Input: part model. Units: mm. Frame: model coordinates. Coordinates: 2 decimals unless noted, no trailing zeros. Write each loop counter-clockwise with the first axis right and the second up, starting at its lowest first coordinate (ties: lowest second). Pieces come first, ordered by that corner, then holes. Notation, with made-up numbers: (-22, -27) -> (35, -27) arc R16 ccw to (35, -22) -> close; hole circle Ø11 at (75.5, -38). An arc over 180 degrees is marked (long way). Use one line per item in the form item = value. Start each with the question number.
(1) Cut plane C-C on y = 0.8. State how many separate pieces and enclosed holes the cut face has, plus the area to 4 significant figures.
(2) Cut plane B-B on z = 8. Return the cut outline in (x, y) (3 decimals).
(3) Ray query, line 1 along X through (y, z) = (0.85, 160); line 2 along Z through (x, y) = (2.5, 0.6); line 3 along X through (y, z) = (1.55, 100). Return the intervals inside material, ascending.
(4) Cut plane A-A on x = 48. Return the cut outline in (y, z) (3 decimals), plus the area to 3 significant figures.
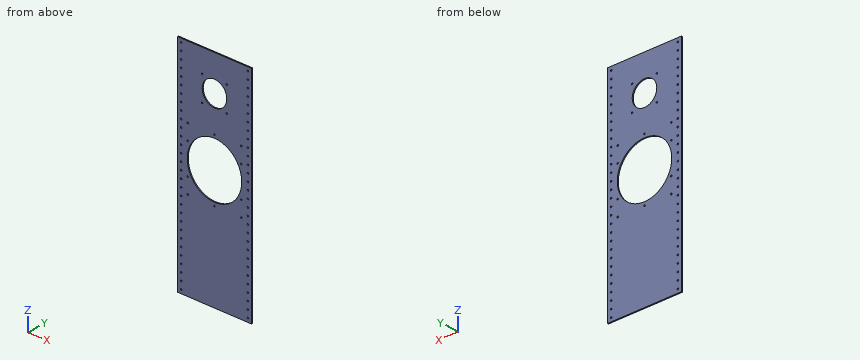
```python
from build123d import *

# Parameters (mm, degrees)
SKETCH1_W           = 204
SKETCH1_H           = 600
SKETCH1_R           = 2.15
SKETCH1_R_2         = 2.125
SKETCH1_R_3         = 33.85
SKETCH1_R_4         = 75.125
BOSS_EXTRUDE1_DEPTH = 3.175


with BuildPart() as part:
    # Sketch1 → Boss-Extrude1 (new body)
    with BuildSketch(Plane(origin=(0, 0, 0), x_dir=(1, 0, 0), z_dir=(0, 1, 0))):
        with Locations((0, -50)):
            Rectangle(SKETCH1_W, SKETCH1_H)
        with Locations(Location((92, 240, 0), (0, 0, 270))):
            Circle(SKETCH1_R, mode=Mode.SUBTRACT)
        with Locations(Location((92, 220, 0), (0, 0, 270))):
            Circle(SKETCH1_R, mode=Mode.SUBTRACT)
        with Locations(Location((92, 200, 0), (0, 0, 270))):
            Circle(SKETCH1_R, mode=Mode.SUBTRACT)
        with Locations(Location((92, 180, 0), (0, 0, 270))):
            Circle(SKETCH1_R, mode=Mode.SUBTRACT)
        with Locations(Location((92, 160, 0), (0, 0, 270))):
            Circle(SKETCH1_R, mode=Mode.SUBTRACT)
        with Locations(Location((92, 140, 0), (0, 0, 270))):
            Circle(SKETCH1_R, mode=Mode.SUBTRACT)
        with Locations(Location((92, 120, 0), (0, 0, 270))):
            Circle(SKETCH1_R, mode=Mode.SUBTRACT)
        with Locations(Location((92, 100, 0), (0, 0, 270))):
            Circle(SKETCH1_R, mode=Mode.SUBTRACT)
        with Locations(Location((92, 80, 0), (0, 0, 270))):
            Circle(SKETCH1_R, mode=Mode.SUBTRACT)
        with Locations(Location((92, 60, 0), (0, 0, 270))):
            Circle(SKETCH1_R, mode=Mode.SUBTRACT)
        with Locations(Location((92, 40, 0), (0, 0, 270))):
            Circle(SKETCH1_R, mode=Mode.SUBTRACT)
        with Locations(Location((92, 20, 0), (0, 0, 270))):
            Circle(SKETCH1_R, mode=Mode.SUBTRACT)
        with Locations(Location((92, 0, 0), (0, 0, 270))):
            Circle(SKETCH1_R, mode=Mode.SUBTRACT)
        with Locations(Location((92, -20, 0), (0, 0, 270))):
            Circle(SKETCH1_R, mode=Mode.SUBTRACT)
        with Locations(Location((92, -40, 0), (0, 0, 270))):
            Circle(SKETCH1_R, mode=Mode.SUBTRACT)
        with Locations(Location((92, -60, 0), (0, 0, 270))):
            Circle(SKETCH1_R, mode=Mode.SUBTRACT)
        with Locations(Location((92, -80, 0), (0, 0, 270))):
            Circle(SKETCH1_R, mode=Mode.SUBTRACT)
        with Locations(Location((92, -100, 0), (0, 0, 270))):
            Circle(SKETCH1_R, mode=Mode.SUBTRACT)
        with Locations(Location((92, -120, 0), (0, 0, 270))):
            Circle(SKETCH1_R, mode=Mode.SUBTRACT)
        with Locations(Location((92, -140, 0), (0, 0, 270))):
            Circle(SKETCH1_R, mode=Mode.SUBTRACT)
        with Locations(Location((92, -160, 0), (0, 0, 270))):
            Circle(SKETCH1_R, mode=Mode.SUBTRACT)
        with Locations(Location((92, -180, 0), (0, 0, 270))):
            Circle(SKETCH1_R, mode=Mode.SUBTRACT)
        with Locations(Location((92, -200, 0), (0, 0, 270))):
            Circle(SKETCH1_R, mode=Mode.SUBTRACT)
        with Locations(Location((92, -220, 0), (0, 0, 270))):
            Circle(SKETCH1_R, mode=Mode.SUBTRACT)
        with Locations(Location((92, -240, 0), (0, 0, 270))):
            Circle(SKETCH1_R, mode=Mode.SUBTRACT)
        with Locations(Location((92, -260, 0), (0, 0, 270))):
            Circle(SKETCH1_R, mode=Mode.SUBTRACT)
        with Locations(Location((92, -280, 0), (0, 0, 270))):
            Circle(SKETCH1_R, mode=Mode.SUBTRACT)
        with Locations(Location((92, -300, 0), (0, 0, 270))):
            Circle(SKETCH1_R, mode=Mode.SUBTRACT)
        with Locations(Location((92, -320, 0), (0, 0, 270))):
            Circle(SKETCH1_R, mode=Mode.SUBTRACT)
        with Locations(Location((92, -340, 0), (0, 0, 270))):
            Circle(SKETCH1_R, mode=Mode.SUBTRACT)
        with Locations(Location((-92, -340, 0), (0, 0, 90))):
            Circle(SKETCH1_R, mode=Mode.SUBTRACT)
        with Locations(Location((-92, -320, 0), (0, 0, 90))):
            Circle(SKETCH1_R, mode=Mode.SUBTRACT)
        with Locations(Location((-92, -300, 0), (0, 0, 90))):
            Circle(SKETCH1_R, mode=Mode.SUBTRACT)
        with Locations(Location((-92, -280, 0), (0, 0, 90))):
            Circle(SKETCH1_R, mode=Mode.SUBTRACT)
        with Locations(Location((-92, -260, 0), (0, 0, 90))):
            Circle(SKETCH1_R, mode=Mode.SUBTRACT)
        with Locations(Location((-92, -240, 0), (0, 0, 90))):
            Circle(SKETCH1_R, mode=Mode.SUBTRACT)
        with Locations(Location((-92, -220, 0), (0, 0, 90))):
            Circle(SKETCH1_R, mode=Mode.SUBTRACT)
        with Locations(Location((-92, -200, 0), (0, 0, 90))):
            Circle(SKETCH1_R, mode=Mode.SUBTRACT)
        with Locations(Location((-92, -180, 0), (0, 0, 90))):
            Circle(SKETCH1_R, mode=Mode.SUBTRACT)
        with Locations(Location((-92, -160, 0), (0, 0, 90))):
            Circle(SKETCH1_R, mode=Mode.SUBTRACT)
        with Locations(Location((-92, -140, 0), (0, 0, 90))):
            Circle(SKETCH1_R, mode=Mode.SUBTRACT)
        with Locations(Location((-92, -120, 0), (0, 0, 90))):
            Circle(SKETCH1_R, mode=Mode.SUBTRACT)
        with Locations(Location((-92, -100, 0), (0, 0, 90))):
            Circle(SKETCH1_R, mode=Mode.SUBTRACT)
        with Locations(Location((-92, -80, 0), (0, 0, 90))):
            Circle(SKETCH1_R, mode=Mode.SUBTRACT)
        with Locations(Location((-92, -60, 0), (0, 0, 90))):
            Circle(SKETCH1_R, mode=Mode.SUBTRACT)
        with Locations(Location((-92, -40, 0), (0, 0, 90))):
            Circle(SKETCH1_R, mode=Mode.SUBTRACT)
        with Locations(Location((-92, -20, 0), (0, 0, 90))):
            Circle(SKETCH1_R, mode=Mode.SUBTRACT)
        with Locations(Location((-92, 0, 0), (0, 0, 90))):
            Circle(SKETCH1_R, mode=Mode.SUBTRACT)
        with Locations(Location((-92, 20, 0), (0, 0, 90))):
            Circle(SKETCH1_R, mode=Mode.SUBTRACT)
        with Locations(Location((-92, 40, 0), (0, 0, 90))):
            Circle(SKETCH1_R, mode=Mode.SUBTRACT)
        with Locations(Location((-92, 60, 0), (0, 0, 90))):
            Circle(SKETCH1_R, mode=Mode.SUBTRACT)
        with Locations(Location((-92, 80, 0), (0, 0, 90))):
            Circle(SKETCH1_R, mode=Mode.SUBTRACT)
        with Locations(Location((-92, 100, 0), (0, 0, 90))):
            Circle(SKETCH1_R, mode=Mode.SUBTRACT)
        with Locations(Location((-92, 120, 0), (0, 0, 90))):
            Circle(SKETCH1_R, mode=Mode.SUBTRACT)
        with Locations(Location((-92, 140, 0), (0, 0, 90))):
            Circle(SKETCH1_R, mode=Mode.SUBTRACT)
        with Locations(Location((-92, 160, 0), (0, 0, 90))):
            Circle(SKETCH1_R, mode=Mode.SUBTRACT)
        with Locations(Location((-92, 180, 0), (0, 0, 90))):
            Circle(SKETCH1_R, mode=Mode.SUBTRACT)
        with Locations(Location((-92, 200, 0), (0, 0, 90))):
            Circle(SKETCH1_R, mode=Mode.SUBTRACT)
        with Locations(Location((-92, 220, 0), (0, 0, 90))):
            Circle(SKETCH1_R, mode=Mode.SUBTRACT)
        with Locations(Location((-92, 240, 0), (0, 0, 90))):
            Circle(SKETCH1_R, mode=Mode.SUBTRACT)
        with Locations(Location((-74, -157.451, 0), (0, 0, 270))):
            Circle(SKETCH1_R_2, mode=Mode.SUBTRACT)
        with Locations(Location((-74, -115.451, 0), (0, 0, 270))):
            Circle(SKETCH1_R_2, mode=Mode.SUBTRACT)
        with Locations(Location((0, -157.451, 0), (0, 0, 270))):
            Circle(SKETCH1_R_2, mode=Mode.SUBTRACT)
        with Locations(Location((74, -157.451, 0), (0, 0, 90))):
            Circle(SKETCH1_R_2, mode=Mode.SUBTRACT)
        with Locations(Location((74, -115.451, 0), (0, 0, 90))):
            Circle(SKETCH1_R_2, mode=Mode.SUBTRACT)
        with Locations(Location((74, -31.451, 0), (0, 0, 270))):
            Circle(SKETCH1_R_2, mode=Mode.SUBTRACT)
        with Locations(Location((74, 10.549, 0), (0, 0, 270))):
            Circle(SKETCH1_R_2, mode=Mode.SUBTRACT)
        with Locations(Location((0, 10.549, 0), (0, 0, 90))):
            Circle(SKETCH1_R_2, mode=Mode.SUBTRACT)
        with Locations(Location((-74, 10.549, 0), (0, 0, 90))):
            Circle(SKETCH1_R_2, mode=Mode.SUBTRACT)
        with Locations(Location((-74, -31.451, 0), (0, 0, 90))):
            Circle(SKETCH1_R_2, mode=Mode.SUBTRACT)
        with Locations(Location((0, -253.451, 0), (0, 0, 270))):
            Circle(SKETCH1_R_3, mode=Mode.SUBTRACT)
        with Locations(Location((0, -73.451, 0), (0, 0, 270))):
            Circle(SKETCH1_R_4, mode=Mode.SUBTRACT)
        with Locations(Location((-34, -287.451, 0), (0, 0, 270))):
            Circle(SKETCH1_R, mode=Mode.SUBTRACT)
        with Locations(Location((34, -287.451, 0), (0, 0, 90))):
            Circle(SKETCH1_R, mode=Mode.SUBTRACT)
        with Locations(Location((34, -219.451, 0), (0, 0, 270))):
            Circle(SKETCH1_R, mode=Mode.SUBTRACT)
        with Locations(Location((-34, -219.451, 0), (0, 0, 90))):
            Circle(SKETCH1_R, mode=Mode.SUBTRACT)
    extrude(amount=BOSS_EXTRUDE1_DEPTH)


solid = part.part
```
Values:
q1.separate_pieces = 1
q1.enclosed_holes = 76
q1.area = 100,000 mm2
q2.outline = (-102, 0) -> (-36.877, 0) -> (-36.877, 3.175) -> (-102, 3.175) -> close; (36.877, 0) -> (102, 0) -> (102, 3.175) -> (36.877, 3.175) -> close
q3.line_1 = -102 to -94.15, -89.85 to 89.85, 94.15 to 102
q3.line_2 = -250 to -1.63, 148.53 to 219.69, 287.21 to 350
q3.line_3 = -102 to -94.15, -89.85 to -70.28, 70.28 to 89.85, 94.15 to 102
q4.outline = (0, -250) -> (3.175, -250) -> (3.175, 15.66) -> (0, 15.66) -> close; (0, 131.242) -> (3.175, 131.242) -> (3.175, 350) -> (0, 350) -> close
q4.area = 1,540 mm2
